Check sheet for the modelled part. Datum: model origin and axes. Units: mm. Face numbers are marked on the shaded views. Coordinates: 2 decimals unless noted, no trailing zeros. Write each loop counter-clockwise with the first axis right and the second up, starting at its lowest first coordinate (ties: lowest second). Pieces come first, ordered by that corner, then holes. Notation, with made-up numbers: M 73.25,42.5 L 98.25,42.5 A10 cw 98.25,60.5 Z; hole C -12.5,-16.75 d6. An arc over 180 degrees is marked long. Answer as CSV lines item,"result". Start each with the question number.
1) Draft check along X on the marked faces 1, 2 and 3. Enter one of: +X half, -X half, draft (parallel to the pull), parting line (faces both ways), or undercut.
2) Section check B-B (x = -2.5). Record the cut outline in (y, z), and give its area (3 significant figures).
3) Section check A-A (x = -27). Record the cut outline in (y, z).
4) Material ranges on L1, parallel to Z at x = -23, y = -2.6; L2, parallel to X at y = -0.9, z = 8.75; L3, parallel to Z at x = 21, y = -0.25, recorded low to high. Write a range as [from, to].
5) Go/stop test with flat-tipped pins: pin 1 Ø0.6 at (x, y) = (1.5, -1) entering from -Z; pin 2 Ø0.6 at (y, z) = (-3, 16) entering from -X; pin 3 Ø2.5 at (x, z) = (5.5, 10.5) entering from -Y. Record where each tip stops, or that it passes through.
from build123d import *

# Parameters (mm, degrees)
F1_DEPTH = 25.4
F2_W     = 12.7390697598
F2_H     = 1.2400867417
F2_W_2   = 12.2317634523
F2_H_2   = 1.4091897756
F2_W_3   = 12.4008655548
F2_W_4   = 12.2881308198
F2_H_3   = 1.2400858104
F3_DEPTH = 63.5


with BuildPart() as f1:
    # F0 (on Top) → F1 (new body)
    with BuildSketch(Plane.XY):
        with BuildLine():
            Line((25.4060197622, -1.4102543581), (25.4060197622, -0.1402543581))
            Line((25.4060197622, -0.1402543581), (-14.7767802378, -0.1402543581))
            ThreePointArc((-14.7767802378, -0.1402543581), (-22.940352015, -2.3026814229), (-31.1039237922, -0.1402543581))
            Line((-31.1039237922, -0.1402543581), (-31.3214249909, -1.3914910378))
            ThreePointArc((-31.3214249909, -1.3914910378), (-23.0576327568, -3.7192286192), (-14.7885782644, -1.4102543581))
            Line((-14.7885782644, -1.4102543581), (25.4060197622, -1.4102543581))
        make_face()
    extrude(amount=F1_DEPTH)

    # F2 (on Front) → F3 (cut, symmetric)
    with BuildSketch(Plane.XZ):
        with BuildLine():
            Line((-10.3737713591, 13.5085717124), (26.4562286409, 13.5085717124))
            Line((26.4562286409, 13.5085717124), (26.7456762769, 26.4659006628))
            Line((26.7456762769, 26.4659006628), (-32.1357277047, 26.4659006628))
            Line((-32.1357277047, 26.4659006628), (-32.1357277047, 18.3892324567))
            Line((-32.1357277047, 18.3892324567), (-18.7555998564, 18.3892324567))
            add(Edge.make_bspline(
                [(-10.3737713591, 13.5085717124), (-11.2232817613, 13.9691896047), (-14.0927804087, 13.3147734099), (-13.8045436235, 15.6054494371), (-16.9112439708, 17.6451656296), (-18.7555998564, 18.3892324567)],
                knots=[0, 0, 0, 0, 0.3348868544, 0.5606693294, 1, 1, 1, 1], degree=3))
        make_face()
        with BuildLine():
            Line((26.1932773025, -2.3347232873), (26.1932773025, 10.4465098237))
            Line((26.1932773025, 10.4465098237), (-10.6367226975, 10.4465098237))
            add(Edge.make_bspline(
                [(-10.6367226975, 10.4465098237), (-11.3411252296, 10.1161423857), (-13.6269139207, 10.7775876683), (-15.2153835526, 6.7761421787), (-16.1896712658, 5.0349102786), (-18.0228203535, 4.3864340605)],
                knots=[0, 0, 0, 0, 0.2928827632, 0.6363136149, 1, 1, 1, 1], degree=3))
            Line((-18.0228203535, 4.3864340605), (-31.7411561322, 4.3864340605))
            Line((-31.7411561322, 4.3864340605), (-32.1357277047, -2.3347232873))
            Line((-32.1357277047, -2.3347232873), (26.1932773025, -2.3347232873))
        make_face()
        with Locations((-25.4207216203, 16.0031258129)):
            Rectangle(F2_W, F2_H)
        with Locations((-25.2234358341, 13.2692987099)):
            Rectangle(F2_W_2, F2_H_2)
        with Locations((-25.3079868853, 10.0563466549)):
            Rectangle(F2_W_3, F2_H_2)
        with Locations((-25.2516195178, 6.8152113818)):
            Rectangle(F2_W_4, F2_H_3)
    extrude(amount=F3_DEPTH, both=True, mode=Mode.SUBTRACT)


solid = f1.part
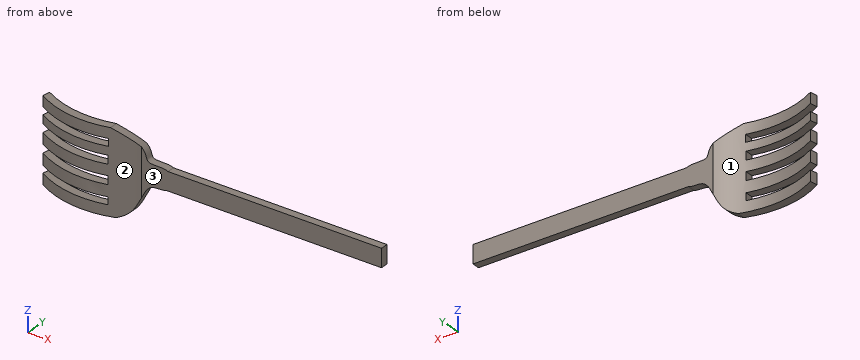
Results found:
1,face 1,"undercut"
1,face 2,"parting line"
1,face 3,"draft"
2,outline,"M -1.41,10.45 L -0.14,10.45 L -0.14,13.51 L -1.41,13.51 Z"
2,area,"3.89 mm2"
3,outline,"M -3.22,4.39 L -1.8,4.39 L -1.8,6.2 L -3.22,6.2 Z; M -3.22,7.44 L -1.8,7.44 L -1.8,9.35 L -3.22,9.35 Z; M -3.22,10.76 L -1.8,10.76 L -1.8,12.56 L -3.22,12.56 Z; M -3.22,13.97 L -1.8,13.97 L -1.8,15.38 L -3.22,15.38 Z; M -3.22,16.62 L -1.8,16.62 L -1.8,18.39 L -3.22,18.39 Z"
4,L1,"z = [4.39, 6.2], [7.44, 9.35], [10.76, 12.56], [13.97, 15.38], [16.62, 18.39]"
4,L2,"x = [-31.24, -29.6], [-16.28, -14.36]"
4,L3,"z = [10.45, 13.51]"
5,pin 1,"stops at z = 10.45"
5,pin 2,"stops at x = -19.05"
5,pin 3,"stops at y = -1.41"
